The model under review builds one solid part; all positions refer to its coordinate system, in mm. Face numbers are marked on the shaded views. Round coordinates to 2 decimals unless told otherwise and drop trailing zeros. Write each loop counter-clockwise with the first axis right and the second up, starting at its lowest first coordinate (ties: lowest second). Pieces come first, ordered by that corner, then holes. Notation, with made-up numbers: (62.5, 25) - (101.5, 25) arc R15 ccw to (101.5, 41) - close; hole circle Ø9 at (28, 34.25). An arc over 180 degrees is marked (long way). Use one line per item in the form item = value.
from build123d import *

# Parameters (mm, degrees)
SKETCH1_W           = 120
SKETCH1_H           = 205
BOSS_EXTRUDE1_DEPTH = 10
BOSS_EXTRUDE2_DEPTH = 5
SKETCH3_W           = 20.5
SKETCH3_H           = 3.5
CUT_EXTRUDE1_DEPTH  = 10
SKETCH4_W           = 20
SKETCH4_H           = 3
BOSS_EXTRUDE3_DEPTH = 10


with BuildPart() as part:
    # Sketch1 → Boss-Extrude1 (new body)
    with BuildSketch(Plane(origin=(0, 0, 0), x_dir=(0, 1, 0), z_dir=(0, 0, 1))):
        Rectangle(SKETCH1_W, SKETCH1_H)
    extrude(amount=BOSS_EXTRUDE1_DEPTH)

    # Sketch2 → Boss-Extrude2 (add)
    with BuildSketch(Plane.XY.offset(10)):
        Polygon((102.5, -60), (97.5, -60), (97.5, 55), (-97.5, 55), (-97.5, -10), (-102.5, -10), (-102.5, 60), (102.5, 60), align=None)
    extrude(amount=BOSS_EXTRUDE2_DEPTH)

    # Sketch3 → Cut-Extrude1 (cut)
    with BuildSketch(Plane(origin=(-102.5, 0, 0), x_dir=(0, -1, 0), z_dir=(-1, 0, 0))):
        with Locations((30, 5)):
            Rectangle(SKETCH3_W, SKETCH3_H)
    extrude(amount=-CUT_EXTRUDE1_DEPTH, mode=Mode.SUBTRACT)

    # Sketch4 → Boss-Extrude3 (add)
    with BuildSketch(Plane.XZ.offset(60)):
        with Locations((-70, 4.996334029)):
            Rectangle(SKETCH4_W, SKETCH4_H)
        with Locations((70, 4.996334029)):
            Rectangle(SKETCH4_W, SKETCH4_H)
    extrude(amount=BOSS_EXTRUDE3_DEPTH)


solid = part.part
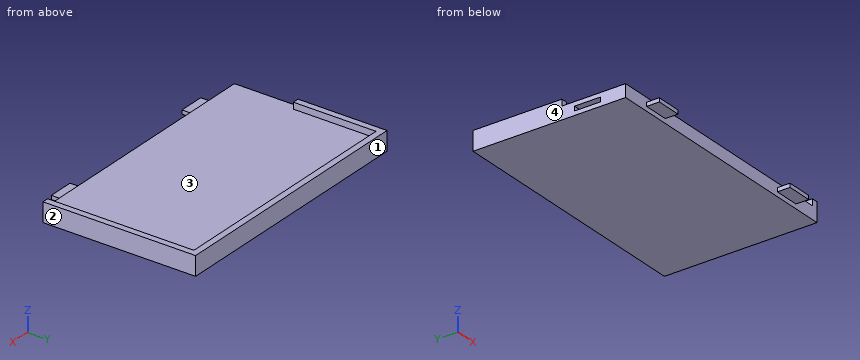
(1) Add section A-A on x = 73.5. Write out the cut boundary in (y, z), then the cut area to 4 significant figures.
Geometry results:
outline = (-70, 3.5) - (-60, 3.5) - (-60, 0) - (60, 0) - (60, 15) - (55, 15) - (55, 10) - (-60, 10) - (-60, 6.5) - (-70, 6.5) - close
area = 1,255 mm2
(2) Add section C-C on z = 12. Write out the cut boundary in (x, y), then the cut area to 4 significant figures.
Geometry results:
outline = (-102.5, -10) - (-97.5, -10) - (-97.5, 55) - (97.5, 55) - (97.5, -60) - (102.5, -60) - (102.5, 60) - (-102.5, 60) - close
area = 1,925 mm2
(3) To check wall thickness, follow L1, parallel to X at y = 31, z = 10.25; L2, parallel to Z at x = 83.5, y = -19.5; L3, parallel to Y at x = -39.5, z = 8.25. State the ranges of each line that lie inside material, in increasing order.
Geometry results:
L1 = -102.5 to -97.5, 97.5 to 102.5
L2 = 0 to 10
L3 = -60 to 60
(4) The part is to be moulded in two halves that separate along X. For the marked faces 1, 2, 3 and 4, say which applies: +X half, -X half, draft (parallel to the pull), parting line (faces both ways), or undercut.
Geometry results:
face_1 = draft
face_2 = +X half
face_3 = undercut
face_4 = -X half
(5) Add section D-D on y = -48.5. Write out the cut boundary in (x, z).
Geometry results:
outline = (-102.5, 0) - (102.5, 0) - (102.5, 15) - (97.5, 15) - (97.5, 10) - (-102.5, 10) - close
(6) Add section B-B on y = 39.5. Write out the cut boundary in (x, z), then the cut area to 3 significant figures.
Geometry results:
outline = (-102.5, 0) - (102.5, 0) - (102.5, 15) - (97.5, 15) - (97.5, 10) - (-97.5, 10) - (-97.5, 15) - (-102.5, 15) - close
area = 2,100 mm2
(7) Insertion check: P1, Ø3, axis at x = -74.5, y = -63.5, coming from the -Z side; P2, Ø1.5, axis at y = -65, z = 4.5, coming from the -X side; P3, Ø4.5, axis at x = -30, z = 9, coming from the -Y side. Each pin has a flat end and moves straight along its axis. Give the tip position at first contact, or say it passes through.
Geometry results:
P1 = 3.5
P2 = -80
P3 = -60
